```python
from build123d import *

# Parameters (mm, degrees)
PAD035_DEPTH         = 10
SKETCH097_W          = 2
SKETCH097_H          = 7.1
POCKET055_DEPTH      = 10.001
POCKET055_DEPTH_BACK = 10.001
SKETCH098_R          = 2.75
POCKET056_DEPTH      = 2.001
POCKET056_DEPTH_BACK = 12.501


with BuildPart() as part:
    # Sketch096 → Pad035 (new body, symmetric)
    with BuildSketch(Plane.XY):
        Polygon((-2, 10), (11, 10), (11, 2.9), (12.5, 2.9), (12.5, -2.9), (11, -2.9), (11, -10), (-2, -10), (-2, -2.9), (0, -2.9), (0, 2.9), (-2, 2.9), align=None)
    extrude(amount=PAD035_DEPTH, both=True)

    # Sketch097 → Pocket055 (cut, two sides)
    with BuildSketch(Plane.XZ) as pocket055_sk:
        with Locations((-1, -6.45)):
            Rectangle(SKETCH097_W, SKETCH097_H)
        with Locations((-1, 6.45)):
            Rectangle(SKETCH097_W, SKETCH097_H)
        Polygon((11, 2.9), (12.5, 4.4), (12.5, -4.4), (11, -2.9), align=None)
    extrude(amount=-POCKET055_DEPTH, mode=Mode.SUBTRACT)
    extrude(pocket055_sk.sketch, amount=POCKET055_DEPTH_BACK, mode=Mode.SUBTRACT)

    # Sketch098 → Pocket056 (cut, two sides)
    with BuildSketch(Plane.YZ) as pocket056_sk:
        Circle(SKETCH098_R)
    extrude(amount=-POCKET056_DEPTH, mode=Mode.SUBTRACT)
    extrude(pocket056_sk.sketch, amount=POCKET056_DEPTH_BACK, mode=Mode.SUBTRACT)


with BuildPart() as part_1:
    # Body022016 placement: moved
    add(part.part.moved(Location((137, 0, -132))))


solid = part_1.part
```
The model under review builds one solid part; all positions refer to its coordinate system, in mm. A direction names the side the tool comes from. Give positions to 0.01 mm unless a question says otherwise; leave off trailing zeros. Write each loop counter-clockwise with the first axis right and the second up, starting at its lowest first coordinate (ties: lowest second). Pieces come first, ordered by that corner, then holes.
(1) To check wall thickness, follow L1, parallel to Y at x = 142, z = -132; L2, parallel to Z at x = 140.75, y = 0; L3, parallel to X at y = 5.75, z = -124. State the ranges of each line that lie inside material, in increasing order.
(2) For P1, Ø3, axis at y = 5.5, z = -127.5, coming from the +X side; P2, Ø2, axis at y = 7.5, z = -126, coming from the -X side; P3, Ø1.6, axis at x = 136, y = 5, coming from the -Z side, all flat-tipped, find the tip position at first contact; note any pin that passes through.
(3) Consider section A-A, the plane z = -132. Give the boundary of the cut face in (x, y), and give its area (3 significant figures).
(4) Consider section C-C, the plane y = 0. Give the boundary of the cut face in (x, z), and give its area (3 significant figures).
(5) The part is to be moulded in two halves that separate along Y. For faces 6 (the flat face through (149, 2.9, -126)), 7 (the flat face through (136, 2.9, -132)), 8 (the flat face through (149.5, 0, -125)), say which applies: released by +Y, released by -Y, zero draft, split by the parting line, or undercut.
(6) Tool access review of faces 1 (the flat face through (136, -2.9, -132)), 2 (the flat face through (136, 6, -129.1)), 3 (the flat face through (149, -2.9, -138)), 4 (the flat face through (148.8, 0, -135.7)), 5 (the flat face through (136, 6, -134.9)): name each direction out of +Z, -Z, +X, -X, +Y, -Y from which nothing blocks a thin tool from reaching the whole face with its end or side.
(7) Consider section B-B, the plane x = 136.5. Give the boundary of the cut face in (y, z), and give its area (3 significant figures).
(8) Consider section D-D, the plane z = -138. Give the boundary of the cut face in (x, y).
Returned:
1. L1: y = -10 to -2.75, 2.75 to 10
1. L2: z = -142 to -134.75, -129.25 to -122
1. L3: x = 137 to 148
2. P1: stops at x = 148
2. P2: stops at x = 137
2. P3: stops at z = -134.9
3. outline: (135, -10) - (148, -10) - (148, -2.75) - (137, -2.75) - (137, -2.9) - (135, -2.9) - close; (135, 2.9) - (137, 2.9) - (137, 2.75) - (148, 2.75) - (148, 10) - (135, 10) - close
3. area: 188 mm2
4. outline: (137, -142) - (149.5, -142) - (149.5, -136.4) - (148, -134.9) - (148, -134.75) - (137, -134.75) - close; (137, -129.25) - (148, -129.25) - (148, -129.1) - (149.5, -127.6) - (149.5, -122) - (137, -122) - close
4. area: 179 mm2
5. face 6: released by +Y
5. face 7: undercut
5. face 8: zero draft
6. face 1: +Z, -Z, -X
6. face 2: +Z, -X, +Y, -Y
6. face 3: +Z, -Z, +X, -Y
6. face 4: +X, +Y, -Y
6. face 5: -Z, -X, +Y, -Y
7. outline: (-10, -134.9) - (-2.9, -134.9) - (-2.9, -129.1) - (-10, -129.1) - close; (2.9, -134.9) - (10, -134.9) - (10, -129.1) - (2.9, -129.1) - close
7. area: 82.4 mm2
8. outline: (137, -10) - (148, -10) - (148, -2.9) - (149.5, -2.9) - (149.5, 2.9) - (148, 2.9) - (148, 10) - (137, 10) - close
